Answer from the drawing. Dimensions are ordinates in mm from the lowest x, y and z of the part. Give positions to 0.01 mm unless a question says otherwise; leave off trailing zeros. Write each loop counter-clockwise with the first axis right and the second up, starting at its lowest first coordinate (ties: lowest second). Pieces come first, ordered by that corner, then holes. Notation, with made-up numbers: M -7,78 L 7,78 A31 cw 7,114 Z; hole C 11.5,52.5 d3. An arc over 180 degrees is marked long. Answer as a JSON object with one key per item and string values.
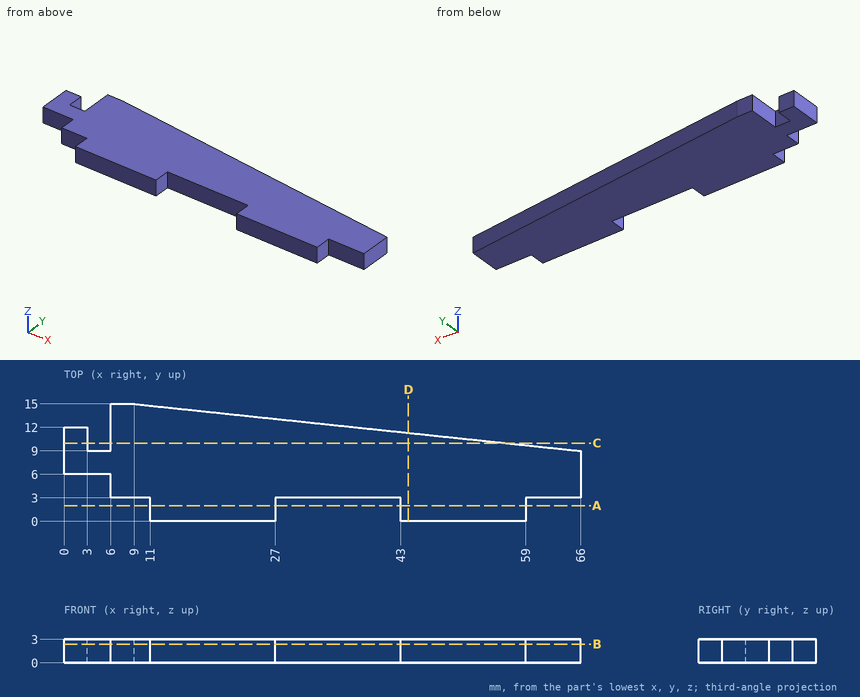
1. A cutting plane is placed at B-B, the plane z = 2.4. Give the vertices of the cut face in (x, y).
Verdict:
{"outline": "M 0,6 L 6,6 L 6,3 L 11,3 L 11,0 L 27,0 L 27,3 L 43,3 L 43,0 L 59,0 L 59,3 L 66,3 L 66,9 L 9,15 L 6,15 L 6,9 L 3,9 L 3,12 L 0,12 Z"}
2. A cutting plane is placed at A-A, the plane y = 2. Give the vertices of the cut face in (x, z).
Verdict:
{"outline": "M 11,0 L 27,0 L 27,3 L 11,3 Z; M 43,0 L 59,0 L 59,3 L 43,3 Z"}
3. A cutting plane is placed at D-D, the plane x = 44. Give the vertices of the cut face in (y, z), plus the area to 3 significant figures.
Verdict:
{"outline": "M 0,0 L 11.32,0 L 11.32,3 L 0,3 Z", "area": "33.9 mm2"}
4. A cutting plane is placed at C-C, the plane y = 10. Give the vertices of the cut face in (x, z), plus the area to 4 significant figures.
Verdict:
{"outline": "M 0,0 L 3,0 L 3,3 L 0,3 Z; M 6,0 L 56.5,0 L 56.5,3 L 6,3 Z", "area": "160.5 mm2"}
5. Flat-ended cylindrical pins translate along their axes: pin 1 (1 mm diameter, centred on y = 4.5, z = 2, fed in from -X); pin 2 (0.9 mm diameter, centred on x = 2, z = 2, fed in from +Y); pin 3 (1.5 mm diameter, centred on x = 4, z = 1.5, fed in from +Y). Find the tip coordinate at first contact, or state that the pin passes through.
Verdict:
{"pin 1": "stops at x = 6", "pin 2": "stops at y = 12", "pin 3": "stops at y = 9"}
6. Consider line 1 along X through (y, z) = (5.25, 2.5); line 2 along Y through (x, z) = (4.5, 0.4); line 3 along Y through (x, z) = (55, 1.9). Determine where each line is inside the solid, lowest interval first.
Verdict:
{"line 1": "x = 6 to 66", "line 2": "y = 6 to 9", "line 3": "y = 0 to 10.16"}
